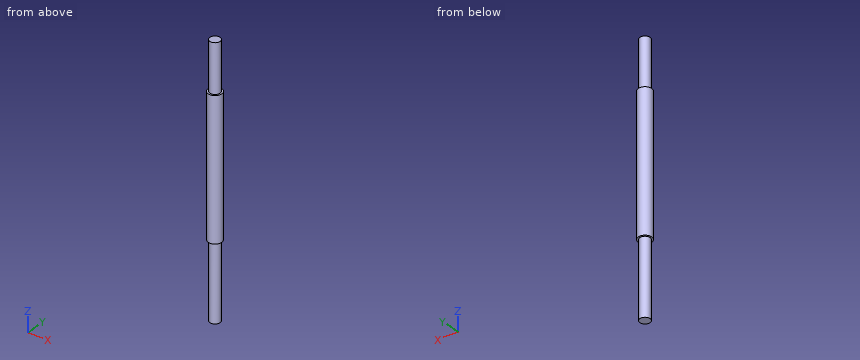
from build123d import *

# Parameters (mm, degrees)
SKETCH1_R           = 6.35
BOSS_EXTRUDE1_DEPTH = 130.3528
SKETCH2_R           = 4.7625
BOSS_EXTRUDE2_DEPTH = 45.466
BOSS_EXTRUDE3_START = 71.12
SKETCH3_R           = 4.7625
BOSS_EXTRUDE3_DEPTH = 71.12


with BuildPart() as part:
    # Sketch1 → Boss-Extrude1 (new body)
    with BuildSketch(Plane.XY):
        Circle(SKETCH1_R)
    extrude(amount=BOSS_EXTRUDE1_DEPTH)

    # Sketch2 → Boss-Extrude2 (add)
    with BuildSketch(Plane.XY.offset(130.3528)):
        with Locations(Location((0, 0, 0), (0, 0, 180))):
            Circle(SKETCH2_R)
    extrude(amount=BOSS_EXTRUDE2_DEPTH)

    # Sketch3 → Boss-Extrude3 (add)
    with BuildSketch(Plane(origin=(0, 0, 0), x_dir=(-1, 0, 0), z_dir=(0, 0, -1)).offset(BOSS_EXTRUDE3_START)):
        Circle(SKETCH3_R)
    extrude(amount=-BOSS_EXTRUDE3_DEPTH)


solid = part.part
Here's how the part is built. I have some questions about the finished solid (model axes, mm). Give positions to 0.01 mm unless a question says otherwise; leave off trailing zeros. Order: outer loops, then holes, each group sorted by start corner. A loop starts at its lowest first (then second) coordinate and runs counter-clockwise, first axis right, second up. Notation, with made-up numbers: M -2,57.25 L 29,57.25 A21 ccw 29,91.25 Z; hole C 40,-32.5 d3. An arc over 180 degrees is marked long. Answer as a JSON object with one key per item and string values. Group by question number.
1) Suppose I cut it at D-D, the plane z = -38.5. Write out the boundary of the cut face in (x, y) (1 decimal).
2) Suppose I cut it at B-B, the plane x = 0. Write out the boundary of the cut face in (y, z).
3) Suppose I cut it at A-A, the plane y = 2.5. Write out the boundary of the cut face in (x, z), plus the area to 3 significant figures.
4) Suppose I cut it at C-C, the plane z = 40.5. Write out the boundary of the cut face in (x, y).
5) I'm going to push flat-ended pins straight in: pin 1 Ø2 at (x, z) = (0.5, 61.5) entering from +Y; pin 2 Ø1 at (y, z) = (-2.5, -38) entering from -X; pin 3 Ø2 at (y, z) = (-2, -40) entering from +X; pin 4 Ø1 at (y, z) = (3, 22) entering from +X. Where does each tip first touch, or does it pass through?
6) Please list where these lines run through material, in increasing order: L1, parallel to Y at x = -0.5, z = 7; L2, parallel to Z at x = -3.5, y = 4; L3, parallel to X at y = -0.75, z = 3.5. Write a range as [from, to].
Results found:
{
 "1": {"outline": "C 0,0 d9.5"},
 "2": {"outline": "M -6.35,0 L -4.76,0 L -4.76,-71.12 L 4.76,-71.12 L 4.76,0 L 6.35,0 L 6.35,130.35 L 4.76,130.35 L 4.76,175.82 L -4.76,175.82 L -4.76,130.35 L -6.35,130.35 Z"},
 "3": {"outline": "M -5.84,0 L -4.05,0 L -4.05,-71.12 L 4.05,-71.12 L 4.05,0 L 5.84,0 L 5.84,130.35 L 4.05,130.35 L 4.05,175.82 L -4.05,175.82 L -4.05,130.35 L -5.84,130.35 Z", "area": "2,470 mm²"},
 "4": {"outline": "C 0,0 d12.7"},
 "5": {"pin 1": "y = 6.35", "pin 2": "x = -4.32", "pin 3": "x = 4.66", "pin 4": "x = 5.84"},
 "6": {"L1": "[-6.33, 6.33]", "L2": "[0, 130.35]", "L3": "[-6.31, 6.31]"}
}
